Work out the finished part from the listing and answer in its coordinate system (mm). A direction names the side the tool comes from. Give positions to 0.01 mm unless a question says otherwise; leave off trailing zeros. Loops run counter-clockwise (first coordinate to the right, second up) from the corner with the lowest first, then second, coordinate; pieces in that order, holes last. Notation, with made-up numbers: (1.5, -6.75) -> (35.5, -6.75) arc R12 cw to (35.5, 13.25) -> close; hole circle Ø9 at (-23.75, 87.25). An arc over 180 degrees is marked (long way). Answer as CSV lines item,"result". Start each with the question number.
1. A tool of negligible diameter and unlimited length cuts with its end or side. For faces 1 (the face through (20.86, -22, -226.01)), 2 (the face through (-27.01, -19.32, 4.27)), 3 (the face through (-28.575, -22, 76)), from which of +Z, -Z, +X, -X, +Y, -Y can it reach the whole face along a straight path? Write none if from no direction.
2. Determine the mould class of faces 4 (the face through (26.965, -18.783, 4.267)), 5 (the face through (-0.311, -22.447, -4.544)), 6 (the face through (-28.575, -22, -76)) for opening direction X: +X half, -X half, draft (parallel to the pull), parting line (faces both ways), or undercut.
3. Flat-ended cylindrical pins translate along their axes: pin 1 Ø0.6 at (x, y) = (-28, -20) entering from -Z (3 decimals); pin 2 Ø1.1 at (x, y) = (-28, -20.5) entering from +Z (3 decimals); pin 3 Ø12 at (y, z) = (-23, 158) entering from -X; pin 4 Ø2.5 at (x, y) = (-28, -22.5) entering from +Z. Find the tip coordinate at first contact, or state that the pin passes through.
4. Find the intervals of material crossed by line 1 along Z through (x, y) = (-22, -25); line 2 along Z through (x, y) = (-24, -25.4); line 3 along Y through (x, z) = (-25.25, -76.2), in increasing order.
5. Find section B-B, the plane x = -13. Give the vertices of the cut face in (y, z) (3 decimals), and give its area (3 significant figures).
from build123d import *

# Parameters (mm, degrees)
BOSS_EXTRUDE1_DEPTH          = 304.8
SHELL1_T                     = -6.35
CUT_EXTRUDE1_DEPTH           = 309.49826681
RIB2_START                   = -22.202989535
RIB2_DEPTH                   = 44.40597907
LPATTERN1_COUNT              = 3
LPATTERN1_PITCH              = 152.4
LPATTERN2_COUNT              = 2
LPATTERN2_PITCH              = 152.4
MIRROR1_COPY_1_DEPTH         = 309.49826681
BOSS_EXTRUDE2_REACH          = 314.443
SKETCH5_W                    = 19.05
SKETCH5_H                    = 25.4
MIRROR4_COPY_1_REACH         = 314.443
MIRROR4_COPY_1_SKETCH_W      = 19.05
MIRROR4_COPY_1_SKETCH_H      = 25.4
F_1_4_20_TAPPED_HOLE1_REACH  = 314.443
F_1_4_20_TAPPED_HOLE1_BORE_R = 2.5527


# Read off the part's stored shape, not the designer's step: Rib2
with BuildPart() as part:
    # Sketch1 → Boss-Extrude1 (new, symmetric)
    with BuildSketch(Plane.XY):
        Polygon((28.575, -38.1), (-28.575, -38.1), (-25.4, 0), (25.4, 0), align=None)
    extrude(amount=BOSS_EXTRUDE1_DEPTH, both=True)

    # Shell1
    shell1_openings = [part.faces().sort_by_distance(p)[0] for p in [
        (0, -38.1, 0),
    ]]
    offset(amount=SHELL1_T, openings=shell1_openings, kind=Kind.INTERSECTION)

    # Sketch2 → Cut-Extrude1 (cut, symmetric)
    with BuildSketch(Plane(origin=(0, 0, 0), x_dir=(1, 0, 0), z_dir=(0, 1, 0))):
        with BuildLine():
            Line((4.7625, -38.1), (4.7625, -114.3))
            ThreePointArc((4.7625, -114.3), (0, -119.0625), (-4.7625, -114.3))
            Line((-4.7625, -114.3), (-4.7625, -38.1))
            ThreePointArc((-4.7625, -38.1), (0, -33.3375), (4.7625, -38.1))
        make_face()
    cut_extrude1 = extrude(amount=CUT_EXTRUDE1_DEPTH, both=True, mode=Mode.SUBTRACT)

    # Rib2 outline → Rib2 (add)
    with BuildSketch(Plane.YZ.offset(RIB2_START)):
        Polygon((-6.35, 146.447234933), (-6.35, 158.352765067), (-38.1, 155.575), (-38.1, 149.225), align=None)
    rib2 = extrude(amount=RIB2_DEPTH)

    # LPattern1: Rib2 ×3
    with Locations(*[(0, 0, -i * LPATTERN1_PITCH) for i in range(1, LPATTERN1_COUNT)]):
        add(rib2)

    # LPattern2: Cut-Extrude1 ×2
    with Locations(*[(0, 0, i * LPATTERN2_PITCH) for i in range(1, LPATTERN2_COUNT)]):
        add(cut_extrude1, mode=Mode.SUBTRACT)

    # Mirror1: Cut-Extrude1 across plane
    add(cut_extrude1.mirror(Plane.XY), mode=Mode.SUBTRACT)

    # Mirror1 copy 1 sketch → Mirror1 copy 1 (cut, symmetric)
    with BuildSketch(Plane(origin=(0, 0, -152.4), x_dir=(1, 0, 0), z_dir=(0, 1, 0))):
        with BuildLine():
            Line((4.7625, 38.1), (4.7625, 114.3))
            ThreePointArc((4.7625, 114.3), (0, 119.0625), (-4.7625, 114.3))
            Line((-4.7625, 114.3), (-4.7625, 38.1))
            ThreePointArc((-4.7625, 38.1), (0, 33.3375), (4.7625, 38.1))
        make_face()
    extrude(amount=MIRROR1_COPY_1_DEPTH, both=True, mode=Mode.SUBTRACT)

    # Sketch5 → Boss-Extrude2 (add, up to next)
    with BuildSketch(Plane(origin=(-28.575, 0, 0), x_dir=(0, 0, -1), z_dir=(1, 0, 0)), mode=Mode.PRIVATE) as boss_extrude2_sk1:
        with Locations((-76.2, -25.4)):
            Rectangle(SKETCH5_W, SKETCH5_H)
    boss_extrude2_tool1 = extrude(boss_extrude2_sk1.sketch, amount=BOSS_EXTRUDE2_REACH, mode=Mode.PRIVATE) - part.part
    boss_extrude2 = boss_extrude2_tool1.solids().sort_by_distance((-28.575, -25.4, 76.2))[0]
    add(boss_extrude2)

    # Mirror2: Boss-Extrude2 across plane
    add(boss_extrude2.mirror(Plane.XY))

    # Mirror3: Boss-Extrude2 across plane
    add(boss_extrude2.mirror(Plane.XY.offset(152.4)))

    # Mirror4 copy 1 sketch → Mirror4 copy 1 (add, up to next)
    with BuildSketch(Plane(origin=(-28.575, 0, -304.8), x_dir=(0, 0, -1), z_dir=(1, 0, 0)), mode=Mode.PRIVATE) as mirror4_copy_1_sk1:
        with Locations((-76.2, -25.4)):
            Rectangle(MIRROR4_COPY_1_SKETCH_W, MIRROR4_COPY_1_SKETCH_H)
    mirror4_copy_1_tool1 = extrude(mirror4_copy_1_sk1.sketch, amount=MIRROR4_COPY_1_REACH, mode=Mode.PRIVATE) - part.part
    add(mirror4_copy_1_tool1.solids().sort_by_distance((-28.575, -25.4, -228.6))[0])

    # 1/4-20 Tapped Hole1 bore → 1/4-20 Tapped Hole1 (cut, up to next)
    with BuildSketch(Plane.ZY.offset(28.575), mode=Mode.PRIVATE) as f_1_4_20_tapped_hole1_sk1:
        with Locations((-228.6, -25.4)):
            Circle(F_1_4_20_TAPPED_HOLE1_BORE_R)
    f_1_4_20_tapped_hole1_tool1 = extrude(f_1_4_20_tapped_hole1_sk1.sketch, amount=-F_1_4_20_TAPPED_HOLE1_REACH, mode=Mode.PRIVATE) & part.part
    # 1/4-20 Tapped Hole1 bore → 1/4-20 Tapped Hole1 (cut, up to next)
    with BuildSketch(Plane.ZY.offset(28.575), mode=Mode.PRIVATE) as f_1_4_20_tapped_hole1_sk2:
        with Locations((-76.2, -25.4)):
            Circle(F_1_4_20_TAPPED_HOLE1_BORE_R)
    f_1_4_20_tapped_hole1_tool2 = extrude(f_1_4_20_tapped_hole1_sk2.sketch, amount=-F_1_4_20_TAPPED_HOLE1_REACH, mode=Mode.PRIVATE) & part.part
    # 1/4-20 Tapped Hole1 bore → 1/4-20 Tapped Hole1 (cut, up to next)
    with BuildSketch(Plane.ZY.offset(28.575), mode=Mode.PRIVATE) as f_1_4_20_tapped_hole1_sk3:
        with Locations((76.2, -25.4)):
            Circle(F_1_4_20_TAPPED_HOLE1_BORE_R)
    f_1_4_20_tapped_hole1_tool3 = extrude(f_1_4_20_tapped_hole1_sk3.sketch, amount=-F_1_4_20_TAPPED_HOLE1_REACH, mode=Mode.PRIVATE) & part.part
    # 1/4-20 Tapped Hole1 bore → 1/4-20 Tapped Hole1 (cut, up to next)
    with BuildSketch(Plane.ZY.offset(28.575), mode=Mode.PRIVATE) as f_1_4_20_tapped_hole1_sk4:
        with Locations((228.6, -25.4)):
            Circle(F_1_4_20_TAPPED_HOLE1_BORE_R)
    f_1_4_20_tapped_hole1_tool4 = extrude(f_1_4_20_tapped_hole1_sk4.sketch, amount=-F_1_4_20_TAPPED_HOLE1_REACH, mode=Mode.PRIVATE) & part.part
    add(f_1_4_20_tapped_hole1_tool1.solids().sort_by_distance((-28.575, -25.4, -228.6))[0], mode=Mode.SUBTRACT)
    add(f_1_4_20_tapped_hole1_tool2.solids().sort_by_distance((-28.575, -25.4, -76.2))[0], mode=Mode.SUBTRACT)
    add(f_1_4_20_tapped_hole1_tool3.solids().sort_by_distance((-28.575, -25.4, 76.2))[0], mode=Mode.SUBTRACT)
    add(f_1_4_20_tapped_hole1_tool4.solids().sort_by_distance((-28.575, -25.4, 228.6))[0], mode=Mode.SUBTRACT)


solid = part.part
Resolved:
1,face 1,"-Y"
1,face 2,"-X, +Y"
1,face 3,"+Z, -Z, -X, +Y, -Y"
2,face 4,"+X half"
2,face 5,"undercut"
2,face 6,"-X half"
3,pin 1,"stops at z = -238.125"
3,pin 2,"stops at z = 238.125"
3,pin 3,"stops at x = -27.82"
3,pin 4,"stops at z = 304.8"
4,line 1,"z = -304.8 to -231.12, -226.08 to -78.72, -73.68 to 73.68, 78.72 to 226.08, 231.12 to 304.8"
4,line 2,"z = -304.8 to -231.15, -226.05 to -78.75, -73.65 to 73.65, 78.75 to 226.05, 231.15 to 304.8"
4,line 3,"y = -38.1 to -27.95, -22.85 to 0"
5,outline,"(-38.1, -304.8) -> (0, -304.8) -> (0, 304.8) -> (-38.1, 304.8) -> (-38.1, 298.45) -> (-6.35, 298.45) -> (-6.35, 158.353) -> (-38.1, 155.575) -> (-38.1, 149.225) -> (-6.35, 146.447) -> (-6.35, 5.953) -> (-38.1, 3.175) -> (-38.1, -3.175) -> (-6.35, -5.953) -> (-6.35, -146.447) -> (-38.1, -149.225) -> (-38.1, -155.575) -> (-6.35, -158.353) -> (-6.35, -298.45) -> (-38.1, -298.45) -> close"
5,area,"5,140 mm^2"
